The drawing under review shows one solid part. Ordinate dimensions are in mm from its lowest x, y, z. A direction names the side the tool comes from. Coordinates: 2 decimals unless noted, no trailing zeros. Loops run counter-clockwise (first coordinate to the right, second up) from the corner with the lowest first, then second, coordinate; pieces in that order, holes last. Notation, with made-up numbers: M 51,59 L 90,59 A18 cw 90,81 Z; hole C -17,32.5 d5. An arc over 180 degrees is marked long. Answer as a JSON object with one key per item and string values. Group by question number.
1. Consider section D-D (y = 4). State the section outline as (x, z) points.
2. Consider section A-A (z = 18.5). State the section outline as (x, y) points.
3. Insertion check: pin 1 (3 mm diameter, centred on y = 44, z = 21, fed in from -X); pin 2 (8 mm diameter, centred on x = 2.5, z = 14, fed in from +Y); pin 3 (11 mm diameter, centred on y = 28.5, z = 2.5, fed in from -X). Each pin has a flat end and moves straight along its axis. Give the tip position at first contact, or say it passes through.
4. To check wall thickness, follow probe 1 along X at (y, z) = (25, 4.5); probe 2 along X at (y, z) = (41, 12); probe 3 along Y at (x, z) = (49.5, 39). State the ranges of each line that lie inside material, in increasing order.
5. Consider section C-C (x = 29.5). State the section outline as (y, z) points.
6. Consider section B-B (y = 45.5). State the section outline as (x, z) points, then the cut area to 3 significant figures.
7. Machinability: for the marked faces 1, 2 and 3, which of the approach directions +Z, -Z, +X, -X, +Y, -Y give a long, thin tool a straight path to every point of the face, cutting with its end or side? Answer none if there is none.
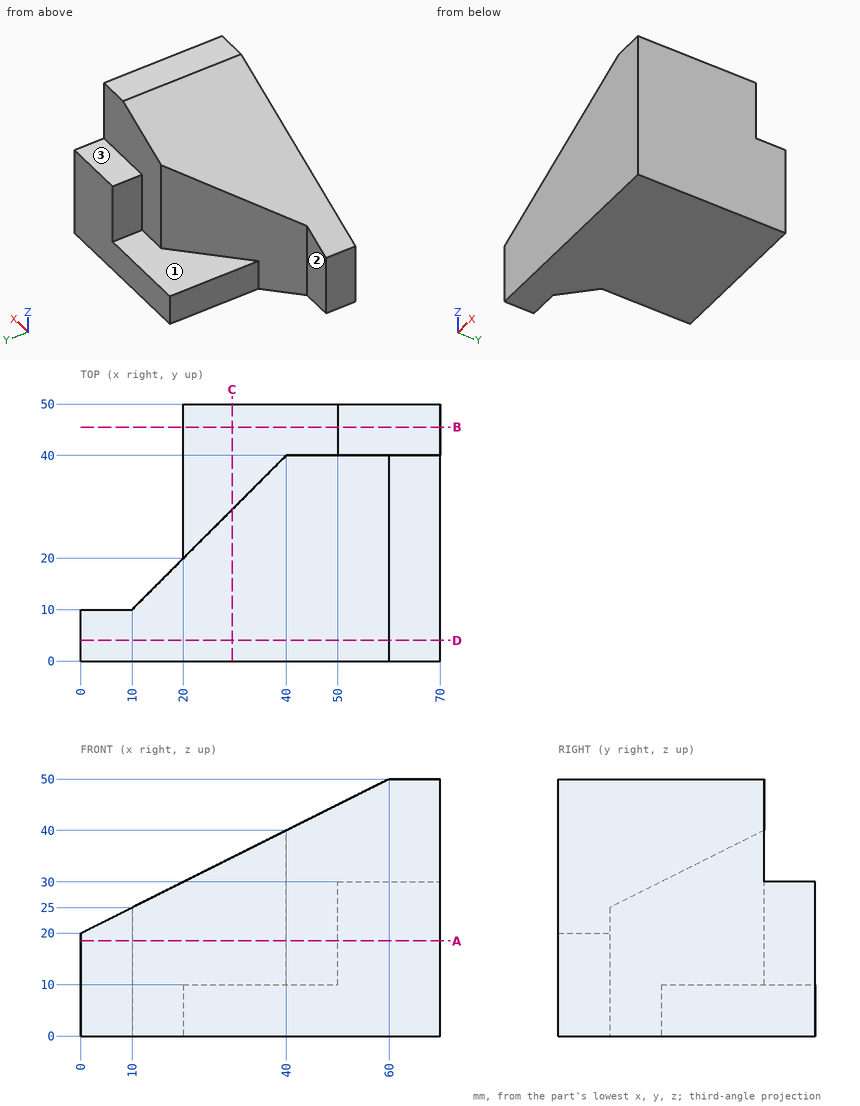
Findings below:
{
 "1": {"outline": "M 0,0 L 70,0 L 70,50 L 60,50 L 0,20 Z"},
 "2": {"outline": "M 0,0 L 70,0 L 70,50 L 50,50 L 50,40 L 40,40 L 10,10 L 0,10 Z"},
 "3": {"pin 1": "stops at x = 50", "pin 2": "stops at y = 10", "pin 3": "stops at x = 20"},
 "4": {"probe 1": "x = 20 to 70", "probe 2": "x = 50 to 70", "probe 3": "y = 0 to 40"},
 "5": {"outline": "M 0,0 L 50,0 L 50,10 L 29.5,10 L 29.5,34.75 L 0,34.75 Z"},
 "6": {"outline": "M 20,0 L 70,0 L 70,30 L 50,30 L 50,10 L 20,10 Z", "area": "900 mm^2"},
 "7": {"face 1": "+Z, -X, +Y", "face 2": "+Z, -Z, -X, +Y", "face 3": "+Z, +X, -X, +Y"}
}
